Part model, mm, in its own coordinate system. A direction names the side the tool comes from. Round coordinates to 2 decimals unless told otherwise and drop trailing zeros. Loops run counter-clockwise (first coordinate to the right, second up) from the corner with the lowest first, then second, coordinate; pieces in that order, holes last. Notation, with made-up numbers: M 70,39.5 L 93,39.5 A34 cw 93,71.5 Z; hole C 45.25,75 d4. An arc over 180 degrees is marked long. Put each result on its own line as item: value. Start each with the question number.
1) Pull direction Z, two halves, no side cores. Call faces 5 (the flat face through (44, -53, 16.7)), 6 (the flat face through (63, -10, 20)): +Z half, -Z half, draft (parallel to the pull), parting line (faces both ways), or undercut.
2) Which spindle directions (+Z, -Z, +X, -X, +Y, -Y) get a long thin tool onto all of the face, cutting with end or side? Do faces 1 (the flat face through (44, -53, 23.3)), 2 (the flat face through (44, -43, 14.5)), 3 (the flat face through (66.15, 0, 20)), 4 (the cylindrical face through (20.55, -43.24, 19.88)). Say none if no direction does.
3) Probe line 1 along Z through (x, y) = (0, -19); line 2 along X through (y, z) = (-33, 4); line 3 along X through (y, z) = (3, 27). List the from-to ranges inside material, lowest first.
4) Slice it at A-A on y = -26. Give the cut face in (x, z).
5) Slice it at D-D on x = 7.5. Give the cut face in (y, z).
6) Slice it at B-B on x = -43. Give the cut face in (y, z), then the cut area to 3 significant figures.
7) Slice it at C-C on z = 20. State how many separate pieces and enclosed holes the cut face has, then the cut area to 3 significant figures.
8) Drop flat-ended pins along their axis: pin 1 Ø13.5 at (y, z) = (-2, 21) entering from -X; pin 2 Ø8 at (y, z) = (1.5, 19.5) entering from +X; pin 3 Ø11 at (y, z) = (2, 28.5) entering from -X. Give the stop position or say it passes through.
```python
from build123d import *

# Parameters (mm, degrees)
SKETCH_1_W                  = 12.3
SKETCH_1_H                  = 7.3
SKETCH_1_W_2                = 7.3
SKETCH_1_H_2                = 12.3
EXTRUDE_1_DEPTH             = 40
CHAMFER_1_SIZE              = 5
CHAMFER_2_SIZE              = 5
CHAMFER_3_SIZE              = 5
SKETCH_25_R                 = 5
CUT_EXTRUDE_1452_DEPTH      = 15
SKETCH_26_R                 = 2.5
CUT_EXTRUDE_1599_DEPTH      = 132.766839531
SKETCH_23_R                 = 5
CUT_EXTRUDE_1755_DEPTH      = 25
CUT_EXTRUDE_1893_REACH      = 219.313
SKETCH_24_R                 = 2.5
MIRROR_2083_COPY_1_SKETCH_R = 5
MIRROR_2083_COPY_1_DEPTH    = 25
MIRROR_2083_COPY_2_REACH    = 219.313
MIRROR_2083_COPY_2_SKETCH_R = 2.5
HOLE_START                  = -60
HOLE_WIZARD_M6_2_DEPTH      = 20
HOLE_START_2                = -46.4
HOLE_WIZARD_M6_2_2_DEPTH    = 6.4


# Read off the part's stored shape, not the designer's step: M6 六角承窩頭蓋螺釘的柱孔2
with BuildPart() as part:
    # 草圖1 → 填料-伸長1 (new body)
    with BuildSketch(Plane.XY):
        Polygon((-82.5, 10), (-47.5, 10), (-47.5, -10), (-77.5, -10), (-77.5, -40), (-10, -40), (-10, 12.5), (10, 12.5), (10, -40), (77.5, -40), (77.5, -10), (47.5, -10), (47.5, 10), (82.5, 10), (102.5, -10), (102.5, -60), (-102.5, -60), (-102.5, -10), align=None)
        with Locations((60, 0)):
            Rectangle(SKETCH_1_W, SKETCH_1_H, mode=Mode.SUBTRACT)
        with Locations((-60, 0)):
            Rectangle(SKETCH_1_W, SKETCH_1_H, mode=Mode.SUBTRACT)
        Rectangle(SKETCH_1_W_2, SKETCH_1_H_2, mode=Mode.SUBTRACT)
    extrude(amount=EXTRUDE_1_DEPTH)

    # 導角1
    chamfer_1_edges = [part.edges().sort_by_distance(p)[0] for p in [
        (-47.5, -10, 20),
        (-10, 12.5, 20),
        (10, 12.5, 20),
        (47.5, -10, 20),
        (47.5, 10, 20),
        (-47.5, 10, 20),
    ]]
    chamfer(chamfer_1_edges, length=CHAMFER_1_SIZE)

    # 導角2
    chamfer_2_edges = [part.edges().sort_by_distance(p)[0] for p in [
        (-77.5, -10, 20),
        (-77.5, -40, 20),
        (-10, -40, 20),
        (10, -40, 20),
        (77.5, -40, 20),
        (77.5, -10, 20),
    ]]
    chamfer(chamfer_2_edges, length=CHAMFER_2_SIZE)

    # 導角3
    chamfer_3_edges = [part.edges().sort_by_distance(p)[0] for p in [
        (102.5, -60, 20),
        (-102.5, -60, 20),
    ]]
    chamfer(chamfer_3_edges, length=CHAMFER_3_SIZE)

    # 草圖25 → Cut-Extrude 1452 (cut)
    with BuildSketch(Plane(origin=(0, -60, 0), x_dir=(-1, 0, 0), z_dir=(0, -1, 0))):
        with Locations(Location((0, -10, 0), (0, 0, 180))):
            Circle(SKETCH_25_R)
    cut_extrude_1452 = extrude(amount=-CUT_EXTRUDE_1452_DEPTH, mode=Mode.SUBTRACT)

    # 草圖26 → Cut-Extrude 1599 (cut, through all)
    with BuildSketch(Plane(origin=(0, -60, 0), x_dir=(-1, 0, 0), z_dir=(0, -1, 0))):
        with Locations(Location((0, -10, 0), (0, 0, 180))):
            Circle(SKETCH_26_R)
    cut_extrude_1599 = extrude(amount=-CUT_EXTRUDE_1599_DEPTH, mode=Mode.SUBTRACT)

    # Mirror 1698: Cut-Extrude 1452, Cut-Extrude 1599 across plane
    add(cut_extrude_1452.mirror(Plane(origin=(0, 0, 20), x_dir=(1, 0, 0), z_dir=(0, 0, -1))), mode=Mode.SUBTRACT)
    add(cut_extrude_1599.mirror(Plane(origin=(0, 0, 20), x_dir=(1, 0, 0), z_dir=(0, 0, -1))), mode=Mode.SUBTRACT)

    # 草圖23 → Cut-Extrude 1755 (cut)
    with BuildSketch(Plane(origin=(102.5, 0, 0), x_dir=(0, 0, -1), z_dir=(1, 0, 0))):
        with Locations(Location((-10, 0, 0), (0, 0, 90))):
            Circle(SKETCH_23_R)
    cut_extrude_1755 = extrude(amount=-CUT_EXTRUDE_1755_DEPTH, mode=Mode.SUBTRACT)

    # Cut-Extrude 1893: up to this face of the body (flat: up to its plane)
    cut_extrude_1893_end = Plane(part.part.faces().sort_by_distance((3.65, 0, 20))[0])
    # 草圖24 → Cut-Extrude 1893 (cut, up to the picked face)
    with BuildSketch(Plane(origin=(102.5, 0, 0), x_dir=(0, 0, -1), z_dir=(1, 0, 0)), mode=Mode.PRIVATE) as cut_extrude_1893_sk1:
        with Locations(Location((-10, 0, 0), (0, 0, 90))):
            Circle(SKETCH_24_R)
    cut_extrude_1893_tool1 = split(extrude(cut_extrude_1893_sk1.sketch, amount=-CUT_EXTRUDE_1893_REACH, mode=Mode.PRIVATE), bisect_by=cut_extrude_1893_end, keep=Keep.BOTH, mode=Mode.PRIVATE)
    cut_extrude_1893 = cut_extrude_1893_tool1.solids().sort_by(Axis((102.5, 0, 10), (-1, 0, 0)))[0]
    add(cut_extrude_1893, mode=Mode.SUBTRACT)

    # Mirror 2006: Cut-Extrude 1755, Cut-Extrude 1893 across plane
    add(cut_extrude_1755.mirror(Plane.ZY), mode=Mode.SUBTRACT)
    add(cut_extrude_1893.mirror(Plane.ZY), mode=Mode.SUBTRACT)

    # Mirror 2083: Cut-Extrude 1755, Cut-Extrude 1893 across plane
    add(cut_extrude_1755.mirror(Plane(origin=(0, 0, 20), x_dir=(1, 0, 0), z_dir=(0, 0, -1))), mode=Mode.SUBTRACT)
    add(cut_extrude_1893.mirror(Plane(origin=(0, 0, 20), x_dir=(1, 0, 0), z_dir=(0, 0, -1))), mode=Mode.SUBTRACT)

    # Mirror 2083 copy 1 sketch → Mirror 2083 copy 1 (cut)
    with BuildSketch(Plane(origin=(-102.5, 0, 40), x_dir=(0, 0, 1), z_dir=(-1, 0, 0))):
        with Locations(Location((-10, 0, 0), (0, 0, 90))):
            Circle(MIRROR_2083_COPY_1_SKETCH_R)
    extrude(amount=-MIRROR_2083_COPY_1_DEPTH, mode=Mode.SUBTRACT)

    # Mirror 2083 copy 2: up to this face of the body (flat: up to its plane)
    mirror_2083_copy_2_end = Plane(part.part.faces().sort_by_distance((-3.65, 0, 20))[0])
    # Mirror 2083 copy 2 sketch → Mirror 2083 copy 2 (cut, up to the picked face)
    with BuildSketch(Plane(origin=(-102.5, 0, 40), x_dir=(0, 0, 1), z_dir=(-1, 0, 0)), mode=Mode.PRIVATE) as mirror_2083_copy_2_sk1:
        with Locations(Location((-10, 0, 0), (0, 0, 90))):
            Circle(MIRROR_2083_COPY_2_SKETCH_R)
    mirror_2083_copy_2_tool1 = split(extrude(mirror_2083_copy_2_sk1.sketch, amount=-MIRROR_2083_COPY_2_REACH, mode=Mode.PRIVATE), bisect_by=mirror_2083_copy_2_end, keep=Keep.BOTH, mode=Mode.PRIVATE)
    add(mirror_2083_copy_2_tool1.solids().sort_by(Axis((-102.5, 0, 30), (1, 0, 0)))[0], mode=Mode.SUBTRACT)

    # M6 六角承窩頭蓋螺釘的柱孔2 outline → M6 六角承窩頭蓋螺釘的柱孔2 (cut)
    with BuildSketch(Plane(origin=(0, 0, 0), x_dir=(1, 0, 0), z_dir=(0, 1, 0)).offset(HOLE_START)):
        with BuildLine():
            Line((26.05, -23.3), (61.45, -23.3))
            ThreePointArc((61.45, -23.3), (64.75, -20), (61.45, -16.7))
            Line((61.45, -16.7), (26.05, -16.7))
            ThreePointArc((26.05, -16.7), (22.75, -20), (26.05, -23.3))
        make_face()
    hole_wizard_m6_2 = extrude(amount=HOLE_WIZARD_M6_2_DEPTH, mode=Mode.SUBTRACT)

    # Hole Wizard M6 _2 2 outline → Hole Wizard M6 _2 2 (cut)
    with BuildSketch(Plane(origin=(0, 0, 0), x_dir=(1, 0, 0), z_dir=(0, 1, 0)).offset(HOLE_START_2)):
        with BuildLine():
            Line((26.05, -25.5), (61.45, -25.5))
            ThreePointArc((61.45, -25.5), (66.95, -20), (61.45, -14.5))
            Line((61.45, -14.5), (26.05, -14.5))
            ThreePointArc((26.05, -14.5), (20.55, -20), (26.05, -25.5))
        make_face()
        with BuildLine():
            ThreePointArc((61.45, -16.7), (64.75, -20), (61.45, -23.3))
            Line((61.45, -23.3), (26.05, -23.3))
            ThreePointArc((26.05, -23.3), (22.75, -20), (26.05, -16.7))
            Line((26.05, -16.7), (61.45, -16.7))
        make_face(mode=Mode.SUBTRACT)
    hole_wizard_m6_2_2 = extrude(amount=HOLE_WIZARD_M6_2_2_DEPTH, mode=Mode.SUBTRACT)

    # Mirror 2781: M6 六角承窩頭蓋螺釘的柱孔2, Hole Wizard M6 _2 2 across plane
    add(hole_wizard_m6_2.mirror(Plane.ZY), mode=Mode.SUBTRACT)
    add(hole_wizard_m6_2_2.mirror(Plane.ZY), mode=Mode.SUBTRACT)


solid = part.part
```
Recorded:
1. face 5: undercut
1. face 6: draft
2. face 1: -Y
2. face 2: none
2. face 3: +Z, -Z
2. face 4: +Y
3. line 1: z = 0 to 7.5, 12.5 to 27.5, 32.5 to 40
3. line 2: x = -102.5 to -77.5, -10 to 10, 77.5 to 102.5
3. line 3: x = -77.5 to -66.15, -53.85 to -47.5, -10 to -3.65, 3.65 to 10, 47.5 to 53.85, 66.15 to 77.5
4. outline: M -102.5,0 L -77.5,0 L -77.5,40 L -102.5,40 Z; M -10,0 L 10,0 L 10,40 L -10,40 Z; M 77.5,0 L 102.5,0 L 102.5,40 L 77.5,40 Z; hole C 0,10 d5; hole C 0,30 d5
5. outline: M -60,0 L 10,0 L 10,40 L -60,40 Z; hole C 0,10 d5; hole C 0,30 d5
6. outline: M -60,0 L -40,0 L -40,14.5 L -46.4,14.5 L -46.4,16.7 L -60,16.7 Z; M -60,23.3 L -46.4,23.3 L -46.4,25.5 L -40,25.5 L -40,40 L -60,40 Z
6. area: 640 mm2
7. separate pieces: 3
7. enclosed holes: 3
7. area: 6,420 mm2
8. pin 1: stops at x = -101.25
8. pin 2: stops at x = 95
8. pin 3: stops at x = -95.34
